Here's how the part is built. I have some questions about the finished solid (model axes, mm). Face numbers are marked on the shaded views. A direction names the side the tool comes from. Coordinates: 2 decimals unless noted, no trailing zeros. Write each loop counter-clockwise with the first axis right and the second up, starting at its lowest first coordinate (ties: lowest second). Pieces come first, ordered by that corner, then holes.
(1) For pin 1 Ø8 at (x, y) = (4, -8) entering from +Z; pin 2 Ø5 at (x, y) = (33.5, 0.5) entering from +Z; pin 3 Ø0.5 at (x, z) = (0.5, 2) entering from -Y; pin 4 Ø4 at (x, y) = (23.5, -5) entering from -Z, each with a flat end and sliding along its axis, tell me the tip position at first contact or that it passes through.
(2) Thinking about a two-plate mould opening in X: for the marked faces 6, 7 and 8, which applies, released by +X, released by -X, zero draft, split by the parting line, or undercut?
(3) Imagine slicing it at C-C, the plane z = 4.75. List the corners of the cut face in (x, y) for me.
(4) Which directions (+Z, -Z, +X, -X, +Y, -Y) give clear straight access to the entire face, cutting with the end or side of a thin tool? Please do the marked faces 1, 2, 3, 4 and 5.
(5) Imagine slicing it at B-B, the plane y = -8. List the corners of the cut face in (x, z) for me.
(6) Please list where these lines run through material, in increasing order: probe 1 along Y at (x, z) = (24.5, -2); probe 2 along X at (y, z) = (-9, 1); probe 3 along Z at (x, y) = (18, -2.25).
(7) Imagine slicing it at D-D, the plane x = 4. List the corners of the cut face in (y, z) for me.
(8) Imagine slicing it at A-A, the plane x = 17.5. List the corners of the cut face in (y, z) for me.
Autodesk Inventor part; units mm, degrees
ref_plane "YZ Plane" through (0, 0, 0) normal (1, 0, 0) x (0, 1, 0)
ref_plane "XZ Plane" through (0, 0, 0) normal (0, 1, 0) x (-1, 0, 0)
ref_plane "XY Plane" through (0, 0, 0) normal (0, 0, 1) x (1, 0, 0)
sketch "스케치1" plane through (0, 0, 0) normal (0, 0, 1) x (1, 0, 0)
  line L0 (0, 0) -> (0, -14)
  line L1 (0, -14) -> (38, -14)
  line L2 (38, -14) -> (38, 4)
  line L3 (38, 4) -> (24, 4)
  line L4 (24, 4) -> (24, 0)
  line L5 (24, 0) -> (0, 0)
  line L6 (8, 0) -> (8, -14)
  dimension "d0" = 18
  dimension "d1" = 38
  dimension "d2" = 14
  dimension "d3" = 14
  dimension "d4" = 8
extrude "돌출1" add sketch "스케치1" along normal mid plane 6 contours L5 L4 L3 L2 L1 L6
extrude "돌출2" add sketch "스케치1" along normal mid plane 16 contours L5 L6 L1 L0
fillet "모깎기1" radius 4 1 edges at (24, 0, 0)
fillet "모깎기2" radius 14 1 edges at (38, -14, 0)
chamfer "모따기1" distance 5 angle 45 1 edges at (0, -14, 0)
chamfer "모따기2" distance 5 angle 45 1 edges at (8, 0, 5.5)
chamfer "모따기3" distance 5 angle 45 1 edges at (8, 0, -5.5)
sketch "스케치2" plane through (0, 0, 8) normal (0, 0, 1) x (1, 0, 0)
  circle A0 centre (4, -8) radius 2.5
  line L0 (0, 0) -> (0, -9)
  line L1 (5, -14) -> (8, -14)
  dimension "d20" = 5
  dimension "d21" = 4
  dimension "d22" = 6
sketch "스케치3" plane through (0, 0, 3) normal (0, 0, 1) x (1, 0, 0)
  line L0 (31, -2) -> (26, -7) construction
  line L1 (28.8787, 0.1213) -> (23.8787, -4.8787)
  line L2 (28.1213, -9.1213) -> (33.1213, -4.1213)
  arc A0 (33.1213, -4.1213) -> (28.8787, 0.1213) centre (31, -2) ccw
  arc A1 (23.8787, -4.8787) -> (28.1213, -9.1213) centre (26, -7) ccw
  line L3 (38, 0) -> (38, 4)
  line L4 (38, 4) -> (24, 4)
  line L5 (26, -7) -> (14, -7) construction
  line L6 (26, -4) -> (14, -4)
  line L7 (14, -10) -> (26, -10)
  arc A2 (26, -10) -> (26, -4) centre (26, -7) ccw
  arc A3 (14, -4) -> (14, -10) centre (14, -7) ccw
  point P0 (0, 0)
  point P1 (28.5, -4.5)
  point P2 (20, -7)
  point P3 (24.7574, -4)
  dimension "d23" = 6
  dimension "d24" = 45
  dimension "d25" = 7
  dimension "d26" = 6
  dimension "d27" = 6
  dimension "d28" = 24
  dimension "d29" = 5
extrude "돌출3" cut sketch "스케치3" against normal blind 16
extrude "돌출4" cut sketch "스케치2" against normal blind 16
sketch "스케치4" plane through (0, 0, -8) normal (-1, 0, 0) x (0, 0, 1)
  line L0 (3.7292, -1.2202) -> (13.2257, -1.2202) construction
  line L1 (13.2257, -1.2202) -> (13.2257, -8.3293) construction
  line L2 (13.2257, -8.3293) -> (3.7292, -8.3293) construction
  line L3 (3.7292, -8.3293) -> (3.7292, -1.2202) construction
  line L4 (7.936, -7.4487) -> (4.1741, -7.4487)
  line L5 (4.1741, -7.4487) -> (4.1741, -6.5837)
  spline S0 degree 2 poles (4.1741, -6.5837) (4.5795, -6.203) (5.3012, -5.4961) (5.6472, -5.1155) knots 0 0 0 1 2 2 2
  spline S1 degree 2 poles (5.6472, -5.1155) (6.3442, -4.3493) (6.8534, -3.4299) (6.8534, -2.9405) knots 0 0 0 1 2 2 2
  spline S2 degree 2 poles (6.8534, -2.9405) (6.8534, -2.6834) (6.6952, -2.2979) (6.5518, -2.1743) knots 0 0 0 1 2 2 2
  spline S3 degree 2 poles (6.5518, -2.1743) (6.4085, -2.0507) (6.0328, -1.9271) (5.8054, -1.9271) knots 0 0 0 1 2 2 2
  spline S4 degree 2 poles (5.8054, -1.9271) (5.5879, -1.9271) (5.143, -2.0359) (4.9403, -2.1199) knots 0 0 0 1 2 2 2
  spline S5 degree 2 poles (4.9403, -2.1199) (4.7673, -2.1891) (4.446, -2.3868) (4.3471, -2.456) knots 0 0 0 1 2 2 2
  line L6 (4.3471, -2.456) -> (4.3027, -2.456)
  line L7 (4.3027, -2.456) -> (4.3027, -1.586)
  spline S6 degree 2 poles (4.3027, -1.586) (4.5548, -1.4624) (5.4594, -1.2202) (5.8647, -1.2202) knots 0 0 0 1 2 2 2
  spline S7 degree 2 poles (5.8647, -1.2202) (6.7199, -1.2202) (7.6839, -2.1248) (7.6839, -2.896) knots 0 0 0 1 2 2 2
  spline S8 degree 2 poles (7.6839, -2.896) (7.6839, -3.2568) (7.5158, -3.8599) (7.3675, -4.117) knots 0 0 0 1 2 2 2
  spline S9 degree 2 poles (7.3675, -4.117) (7.2192, -4.3839) (6.7891, -4.9079) (6.5518, -5.16) knots 0 0 0 1 2 2 2
  spline S10 degree 2 poles (6.5518, -5.16) (6.1663, -5.5802) (5.2221, -6.4799) (4.9403, -6.7419) knots 0 0 0 1 2 2 2
  line L8 (4.9403, -6.7419) -> (7.936, -6.7419)
  line L9 (7.936, -6.7419) -> (7.936, -7.4487)
  line L10 (12.207, -7.4487) -> (9.2311, -7.4487)
  line L11 (9.2311, -7.4487) -> (9.2311, -6.8259)
  line L12 (9.2311, -6.8259) -> (10.3384, -6.8259)
  line L13 (10.3384, -6.8259) -> (10.3384, -2.7378)
  line L14 (10.3384, -2.7378) -> (9.2311, -2.7378)
  line L15 (9.2311, -2.7378) -> (9.2311, -2.1792)
  spline S11 degree 2 poles (9.2311, -2.1792) (9.8589, -2.1792) (10.4521, -1.8233) (10.4916, -1.329) knots 0 0 0 1 2 2 2
  line L16 (10.4916, -1.329) -> (11.1244, -1.329)
  line L17 (11.1244, -1.329) -> (11.1244, -6.8259)
  line L18 (11.1244, -6.8259) -> (12.207, -6.8259)
  line L19 (12.207, -6.8259) -> (12.207, -7.4487)
  point P0 (8, 0)
extrude "돌출5" cut sketch "스케치4" against normal blind 1
properties part number "1번부품"
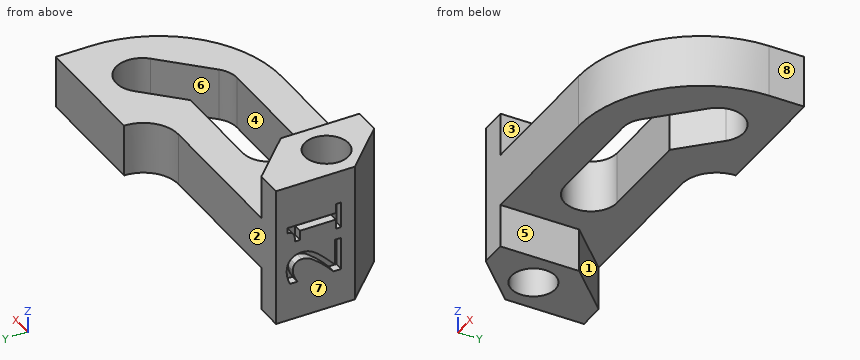
Recorded:
1. pin 1: stops at z = 8
1. pin 2: stops at z = 3
1. pin 3: stops at y = -9.75
1. pin 4: stops at z = -3
2. face 6: undercut
2. face 7: released by -X
2. face 8: released by +X
3. outline: (0, -9) - (5, -14) - (8, -14) - (8, -5) - (3, 0) - (0, 0) - close; hole circle Ø5 at (4, -8)
4. face 1: -Z, +X, +Y
4. face 2: +Z, -Z, -X, +Y
4. face 3: +Z, +X, +Y, -Y
4. face 4: +Z, -Z
4. face 5: -Z, +X, +Y, -Y
5. outline: (0, -8) - (1.5, -8) - (1.5, 8) - (0, 8) - close; (6.5, -8) - (8, -8) - (8, -3) - (11.17, -3) - (11.17, 3) - (8, 3) - (8, 8) - (6.5, 8) - close; (29.24, -3) - (35.49, -3) - (35.49, 3) - (29.24, 3) - close
6. probe 1: y = -13.99 to -10, -4 to 4
6. probe 2: x = 0 to 1.71, 6.29 to 11.76, 28.24 to 34.72
6. probe 3: z = -3 to 3
7. outline: (-13, -8) - (-10.5, -8) - (-10.5, 8) - (-13, 8) - close; (-5.5, -8) - (-1, -8) - (-1, -3) - (0, -3) - (0, 3) - (-1, 3) - (-1, 8) - (-5.5, 8) - close
8. outline: (-14, -3) - (-10, -3) - (-10, 3) - (-14, 3) - close; (-4, -3) - (0, -3) - (0, 3) - (-4, 3) - close
